```python
from build123d import *

# Parameters (mm, degrees)
SKETCH1_W                               = 99.5
SKETCH1_H                               = 44
BOSS_EXTRUDE1_DEPTH                     = 6
SKETCH5_R                               = 12.3
CUT_EXTRUDE1_DEPTH                      = 6
SKETCH5_5_R                             = 12.3
CUT_EXTRUDE4_DEPTH                      = 6
SKETCH2_R                               = 1.75
CUT_EXTRUDE8_DEPTH                      = 6
BOSS_EXTRUDE5_START                     = 3
SKETCH2_15_W                            = 7.5
SKETCH2_15_H                            = 44
SKETCH2_15_R                            = 1.75
BOSS_EXTRUDE5_DEPTH                     = 3
BOSS_EXTRUDE6_DEPTH                     = 3
SKETCH8_W                               = 1.4
SKETCH8_H                               = 44
BOSS_EXTRUDE7_DEPTH                     = 0.8
MOVE_FACE3_BY                           = 2
SKETCH9_W                               = 1.4
SKETCH9_H                               = 44
BOSS_EXTRUDE8_DEPTH                     = 0.8
SKETCH12_R                              = 0.875
CUT_EXTRUDE13_DEPTH                     = 44
SKETCH14_R                              = 1.3
CUT_EXTRUDE15_DEPTH                     = 6.5
SKETCH15_R                              = 1.6
CUT_EXTRUDE17_DEPTH                     = 4
SKETCH17_R                              = 1.3
CUT_EXTRUDE18_DEPTH                     = 5.8
SKETCH18_R                              = 1.6
CUT_EXTRUDE19_DEPTH                     = 4
CBORE_FOR_M5_HEX_HEAD_BOLT1_D           = 2.6
CBORE_FOR_M5_HEX_HEAD_BOLT1_CBORE_D     = 3.2
CBORE_FOR_M5_HEX_HEAD_BOLT1_CBORE_DEPTH = 4


with BuildPart() as part:
    # Sketch1 → Boss-Extrude1 (new body)
    with BuildSketch(Plane.XY):
        with Locations((12.809190031, 1.12305296)):
            Rectangle(SKETCH1_W, SKETCH1_H)
    extrude(amount=BOSS_EXTRUDE1_DEPTH)

    # Sketch5 → Cut-Extrude1 (cut)
    with BuildSketch(Plane(origin=(0, 0, 0), x_dir=(-1, 0, 0), z_dir=(0, 0, -1))):
        with Locations(Location((-32.609190031, 1.12305296, 0), (0, 0, 180))):
            Circle(SKETCH5_R)
    extrude(amount=-CUT_EXTRUDE1_DEPTH, mode=Mode.SUBTRACT)

    # Sketch5_5 → Cut-Extrude4 (cut)
    with BuildSketch(Plane(origin=(0, 0, 0), x_dir=(-1, 0, 0), z_dir=(0, 0, -1))):
        with Locations((6.990809969, 1.12305296)):
            Circle(SKETCH5_5_R)
        with Locations(Location((-32.609190031, 1.12305296, 0), (0, 0, 180))):
            Circle(SKETCH5_5_R)
    extrude(amount=-CUT_EXTRUDE4_DEPTH, mode=Mode.SUBTRACT)

    # Sketch2 → Cut-Extrude8 (cut)
    with BuildSketch(Plane.XY.offset(6)):
        with Locations((-33.190809969, 19.37305296)):
            Circle(SKETCH2_R)
        with Locations(Location((58.809190031, 19.37305296, 0), (0, 0, 180))):
            Circle(SKETCH2_R)
        with Locations((58.809190031, -17.12694704)):
            Circle(SKETCH2_R)
        with Locations(Location((-33.190809969, -17.12694704, 0), (0, 0, 180))):
            Circle(SKETCH2_R)
    extrude(amount=-CUT_EXTRUDE8_DEPTH, mode=Mode.SUBTRACT)

    # Sketch2_15 → Boss-Extrude5 (add)
    # profile 1 of 2: a face of its own
    with BuildSketch(Plane.XY.offset(6).offset(BOSS_EXTRUDE5_START)):
        with Locations((-33.190809969, 1.12305296)):
            Rectangle(SKETCH2_15_W, SKETCH2_15_H)
        with Locations((-33.190809969, 19.37305296)):
            Circle(SKETCH2_15_R, mode=Mode.SUBTRACT)
        with Locations(Location((-33.190809969, -17.12694704, 0), (0, 0, 180))):
            Circle(SKETCH2_15_R, mode=Mode.SUBTRACT)
    # profile 2 of 2: a face of its own
    with BuildSketch(Plane.XY.offset(6).offset(BOSS_EXTRUDE5_START)):
        with Locations((58.809190031, 1.12305296)):
            Rectangle(SKETCH2_15_W, SKETCH2_15_H)
        with Locations(Location((58.809190031, 19.37305296, 0), (0, 0, 180))):
            Circle(SKETCH2_15_R, mode=Mode.SUBTRACT)
        with Locations((58.809190031, -17.12694704)):
            Circle(SKETCH2_15_R, mode=Mode.SUBTRACT)
    extrude(amount=-BOSS_EXTRUDE5_DEPTH)

    # Sketch6 → Boss-Extrude6 (add)
    with BuildSketch(Plane.XY.offset(6)):
        with BuildLine():
            Line((11.559190031, -20.87694704), (14.059190031, -20.87694704))
            Line((14.059190031, -20.87694704), (23.329238523, -20.87694704))
            Line((23.329238523, -20.87694704), (23.329238523, -15.22694704))
            ThreePointArc((23.329238523, -15.22694704), (17.186408911, -9.627659693), (14.058246659, -1.92694704))
            Line((14.058246659, -1.92694704), (14.058246659, 4.17305296))
            ThreePointArc((14.058246659, 4.17305296), (17.186408911, 11.873765612), (23.329238523, 17.47305296))
            Line((23.329238523, 17.47305296), (23.329238523, 23.12305296))
            Line((23.329238523, 23.12305296), (14.059190031, 23.12305296))
            Line((14.059190031, 23.12305296), (11.559190031, 23.12305296))
            Line((11.559190031, 23.12305296), (2.28914154, 23.12305296))
            Line((2.28914154, 23.12305296), (2.28914154, 17.47305296))
            ThreePointArc((2.28914154, 17.47305296), (8.431971151, 11.873765612), (11.560133403, 4.17305296))
            Line((11.560133403, 4.17305296), (11.560133403, -1.92694704))
            ThreePointArc((11.560133403, -1.92694704), (8.431971151, -9.627659693), (2.28914154, -15.22694704))
            Line((2.28914154, -15.22694704), (2.28914154, -20.87694704))
            Line((2.28914154, -20.87694704), (11.559190031, -20.87694704))
        make_face()
    extrude(amount=BOSS_EXTRUDE6_DEPTH)

    # Sketch8 → Boss-Extrude7 (add)
    with BuildSketch(Plane.XY.offset(6)):
        with Locations((-27.240809969, 1.12305296)):
            Rectangle(SKETCH8_W, SKETCH8_H)
    extrude(amount=BOSS_EXTRUDE7_DEPTH)

    # Move Face3: a face moved outward by 2.0
    extrude(part.faces().sort_by_distance((12.809190031, 1.12305296, 0))[0], amount=MOVE_FACE3_BY, dir=(0, 0, -1))

    # Sketch9 → Boss-Extrude8 (add)
    with BuildSketch(Plane.XY.offset(6)):
        with Locations((52.859190031, 1.12305296)):
            Rectangle(SKETCH9_W, SKETCH9_H)
    extrude(amount=BOSS_EXTRUDE8_DEPTH)

    # Sketch12 → Cut-Extrude13 (cut)
    with BuildSketch(Plane(origin=(0, 23.12305296, 0), x_dir=(1, 0, 0), z_dir=(0, 1, 0))):
        with Locations(Location((12.809190031, -3, 0), (0, 0, 270))):
            Circle(SKETCH12_R)
        with Locations(Location((12.809190031, -6, 0), (0, 0, 270))):
            Circle(SKETCH12_R)
    extrude(amount=-CUT_EXTRUDE13_DEPTH, mode=Mode.SUBTRACT)

    # Sketch14 → Cut-Extrude15 (cut)
    with BuildSketch(Plane(origin=(0, 0, -2), x_dir=(-1, 0, 0), z_dir=(0, 0, -1))):
        with Locations((-12.809190031, 18.12305296)):
            Circle(SKETCH14_R)
        with Locations((-12.809190031, 12.12305296)):
            Circle(SKETCH14_R)
    extrude(amount=-CUT_EXTRUDE15_DEPTH, mode=Mode.SUBTRACT)

    # Sketch15 → Cut-Extrude17 (cut)
    with BuildSketch(Plane(origin=(0, 0, -2), x_dir=(-1, 0, 0), z_dir=(0, 0, -1))):
        with Locations((-12.809190031, 18.12305296)):
            Circle(SKETCH15_R)
        with Locations((-12.809190031, 12.12305296)):
            Circle(SKETCH15_R)
    extrude(amount=-CUT_EXTRUDE17_DEPTH, mode=Mode.SUBTRACT)

    # Sketch17 → Cut-Extrude18 (cut)
    with BuildSketch(Plane(origin=(0, 0, -2), x_dir=(-1, 0, 0), z_dir=(0, 0, -1))):
        with Locations((-12.809190031, 4.12305296)):
            Circle(SKETCH17_R)
        with Locations((-12.809190031, -1.87694704)):
            Circle(SKETCH17_R)
    extrude(amount=-CUT_EXTRUDE18_DEPTH, mode=Mode.SUBTRACT)

    # Sketch18 → Cut-Extrude19 (cut)
    with BuildSketch(Plane(origin=(0, 0, -2), x_dir=(-1, 0, 0), z_dir=(0, 0, -1))):
        with Locations((-12.809190031, 4.12305296)):
            Circle(SKETCH18_R)
        with Locations((-12.809190031, -1.87694704)):
            Circle(SKETCH18_R)
    extrude(amount=-CUT_EXTRUDE19_DEPTH, mode=Mode.SUBTRACT)

    # CBORE for M5 Hex Head Bolt1 (through all)
    with Locations(Plane(origin=(45.359190031, -16.87694704, -2), x_dir=(-1, 0, 0), z_dir=(0, 0, -1))):
        with Locations((0, 0), (25.5, 0), (39.6, 0), (65.1, 0)):
            CounterBoreHole(CBORE_FOR_M5_HEX_HEAD_BOLT1_D / 2, CBORE_FOR_M5_HEX_HEAD_BOLT1_CBORE_D / 2, CBORE_FOR_M5_HEX_HEAD_BOLT1_CBORE_DEPTH)


solid = part.part
```
CAD build for the part. Positions are in the model's coordinates, mm. A direction names the side the tool comes from. Round coordinates to 2 decimals unless told otherwise and drop trailing zeros. Return JSON: item names as keys, results as strings. Group by question number.
Q1. Band-saw the part on A-A on y = -6. Give the number of separate pieces and of enclosed holes in the cut face, plus the area to 3 significant figures.
Q2. Drill centre lines: line 1 along X through (y, z) = (-5.5, 3.75); line 2 along X through (y, z) = (-1.5, 6.5); line 3 along X through (y, z) = (9.5, -1). Where is each one in solid material? Low to high. Write a range as [from, to].
Q3. Flat gauge pins, fed straight in: pin 1 Ø12 at (x, y) = (-7, -15) entering from +Z; pin 2 Ø1 at (x, y) = (12, -1.5) entering from -Z; pin 3 Ø3.5 at (x, y) = (12.5, 17.5) entering from -Z. Where does each tip first touch, or does it go through?
Q4. Two-plate mould, pull along X, no slides. Class faces 1 (the face through (43.83, -16.4, -0.03)), 2 (the face through (12, 23.123, 2)), 3 (the face through (62.559, 1, 4)), 4 (the face through (-34.481, 20.556, 3.577)): +X half, -X half, draft (parallel to the pull), parting line (faces both ways), or undercut.
Q5. Tool access for faces 5 (the face through (55.059, 1, 8)), 6 (the face through (11.33, -2.49, -0.03)), 7 (the face through (17.12, 11.78, 7.48)), 8 (the face through (12.848, 21.132, 2.126)): list every direction of +Z, -Z, +X, -X, +Y, -Y with a clear straight run to the whole face (end or side of a thin tool).
Solutions:
{
 "1": {"separate pieces": "3", "enclosed holes": "2", "area": "532 mm^2"},
 "2": {"line 1": "x = [-36.94, -17.36], [3.37, 12.36], [13.26, 22.24], [42.97, 62.56]", "line 2": "x = [-36.94, -29.44], [-27.94, -26.54], [11.56, 12.09], [13.53, 14.06], [52.16, 53.56], [55.06, 62.56]", "line 3": "x = [-36.94, -16], [2.02, 23.6], [41.62, 62.56]"},
 "3": {"pin 1": "stops at z = 6", "pin 2": "stops at z = 2", "pin 3": "stops at z = -2"},
 "4": {"face 1": "undercut", "face 2": "draft", "face 3": "+X half", "face 4": "undercut"},
 "5": {"face 5": "+Z, +Y, -Y", "face 6": "-Z", "face 7": "+Z", "face 8": "+Y, -Y"}
}
